Could you check a few things on this model? Use its own coordinates, in mm. Coordinates: 2 decimals unless noted, no trailing zeros. Order: outer loops, then holes, each group sorted by start corner. A loop starts at its lowest first (then second) coordinate and runs counter-clockwise, first axis right, second up. Notation, with made-up numbers: (44.25, 76) - (101.25, 76) arc R26 ccw to (101.25, 101) - close; hole circle Ø7 at (-1.75, 83). An arc over 180 degrees is marked (long way). One line per item, written item: value.
from build123d import *

# Parameters (mm, degrees)
SKETCH1_W           = 35
SKETCH1_H           = 25
SKETCH1_R           = 6.5
SKETCH1_R_2         = 1.5
BOSS_EXTRUDE1_DEPTH = 1.5875
FILLET1_R           = 5


with BuildPart() as part:
    # Sketch1 → Boss-Extrude1 (new body)
    with BuildSketch(Plane.XY):
        with Locations((17.5, 12.5)):
            Rectangle(SKETCH1_W, SKETCH1_H)
        with Locations((17.5, 12.5)):
            Circle(SKETCH1_R, mode=Mode.SUBTRACT)
        with Locations((5, 20)):
            Circle(SKETCH1_R_2, mode=Mode.SUBTRACT)
        with Locations((5, 5)):
            Circle(SKETCH1_R_2, mode=Mode.SUBTRACT)
        with Locations(Location((30, 5, 0), (0, 0, 180))):
            Circle(SKETCH1_R_2, mode=Mode.SUBTRACT)
        with Locations(Location((30, 20, 0), (0, 0, 180))):
            Circle(SKETCH1_R_2, mode=Mode.SUBTRACT)
    extrude(amount=BOSS_EXTRUDE1_DEPTH)

    # Fillet1
    fillet1_edges = [part.edges().sort_by_distance(p)[0] for p in [
        (0, 0, 0.79375),
        (0, 25, 0.79375),
        (35, 25, 0.79375),
        (35, 0, 0.79375),
    ]]
    fillet(fillet1_edges, radius=FILLET1_R)


solid = part.part
Item 1: I want a section at C-C on x = 12.5. Please give me the cut outline in (y, z).
Conclusion:
outline: (0, 0) - (8.35, 0) - (8.35, 1.59) - (0, 1.59) - close; (16.65, 0) - (25, 0) - (25, 1.59) - (16.65, 1.59) - close
Item 2: I want a section at A-A on z = 0.4. Please give me the cut outline in (x, y), then the cut area to 3 significant figures.
Conclusion:
outline: (0, 5) arc R5 ccw to (5, 0) - (30, 0) arc R5 ccw to (35, 5) - (35, 20) arc R5 ccw to (30, 25) - (5, 25) arc R5 ccw to (0, 20) - close; hole circle Ø3 at (5, 5); hole circle Ø3 at (5, 20); hole circle Ø13 at (17.5, 12.5); hole circle Ø3 at (30, 5); hole circle Ø3 at (30, 20)
area: 693 mm²
Item 3: I want a section at D-D on y = 4.5. Please give me the cut outline in (x, z), then the cut area to 3 significant figures.
Conclusion:
outline: (0.03, 0) - (3.59, 0) - (3.59, 1.59) - (0.03, 1.59) - close; (6.41, 0) - (28.59, 0) - (28.59, 1.59) - (6.41, 1.59) - close; (31.41, 0) - (34.97, 0) - (34.97, 1.59) - (31.41, 1.59) - close
area: 46.5 mm²
Item 4: If I drill on probe 1 along Y at (x, z) = (30, 1.15); probe 2 along Y at (x, z) = (20, 0.3); probe 3 along X at (y, z) = (20.5, 1.25), over which ranges is the centre line in solid material (lowest first)?
Conclusion:
probe 1: 0 to 3.5, 6.5 to 18.5, 21.5 to 25
probe 2: 0 to 6.5, 18.5 to 25
probe 3: 0.03 to 3.59, 6.41 to 28.59, 31.41 to 34.97
Item 5: Thinking about a two-plate mould opening in X: for faces 1 (the face through (4.805, 21.487, 0.783)), 2 (the face through (1, 2, 1)), 3 (the face through (17, 25, 1)), which applies, pulls with the +X half, pulls with the -X half, needs draft (parallel to the pull), parting line crosses it, or undercut?
Conclusion:
face 1: undercut
face 2: pulls with the -X half
face 3: needs draft
Item 6: I want a section at B-B on y = 14. Please give me the cut outline in (x, z).
Conclusion:
outline: (0, 0) - (11.18, 0) - (11.18, 1.59) - (0, 1.59) - close; (23.82, 0) - (35, 0) - (35, 1.59) - (23.82, 1.59) - close
